from build123d import *

# Parameters (mm, degrees)
EXTRU_MINCE1_DEPTH      = 16.5
ENL_V_MAT_EXTRU_5_DEPTH = 37.379072455
BOSS_EXTRU_1_DEPTH      = 5
ESQUISSE2_R             = 1.6
ENL_V_MAT_EXTRU_1_DEPTH = 23.509707076
ESQUISSE3_R             = 1.6
ENL_V_MAT_EXTRU_2_DEPTH = 23.509707076
ENL_V_START             = -3
ENL_V_MAT_EXTRU_3_DEPTH = 20.509707076
ENL_V_MAT_EXTRU_4_DEPTH = 20.509707076
CHANFREIN1_SIZE         = 10
CONG_1_R                = 2


with BuildPart() as part:
    # Esquisse1 → Extru.-Mince1 (new, symmetric)
    with BuildSketch(Plane(origin=(0, 0, 0), x_dir=(0, 0, -1), z_dir=(1, 0, 0))):
        Polygon((11, 0), (0, 0), (-8.191520443, -5.735764364), (-4.750061825, -10.650676629), (1.891792733, -6), (11, -6), align=None)
    extrude(amount=EXTRU_MINCE1_DEPTH, both=True)

    # Esquisse7 → Enlèv. mat.-Extru.5 (cut, through all)
    with BuildSketch(Plane.ZY.offset(16.5)):
        Polygon((-1.891792733, -6), (5.081994449, -6), (7.04436757, -7.374068452), (4.750061825, -10.650676629), align=None)
    extrude(amount=-ENL_V_MAT_EXTRU_5_DEPTH, mode=Mode.SUBTRACT)

    # Esquisse6 → Boss.-Extru.1 (add, symmetric)
    with BuildSketch(Plane(origin=(0, 0, 0), x_dir=(0, 0, -1), z_dir=(1, 0, 0))):
        Polygon((1.891792733, -6), (11, -6), (-4.750061825, -10.650676629), (-8.191520443, -5.735764364), (-5.081994449, -6), align=None)
    extrude(amount=BOSS_EXTRU_1_DEPTH, both=True)

    # Esquisse2 → Enlèv. mat.-Extru.1 (cut, through all)
    with BuildSketch(Plane(origin=(0, 0, 0), x_dir=(1, 0, 0), z_dir=(0, 1, 0))):
        with Locations(Location((-12, 6.5, 0), (0, 0, 270))):
            Circle(ESQUISSE2_R)
        with Locations(Location((12, 6.5, 0), (0, 0, 90))):
            Circle(ESQUISSE2_R)
    extrude(amount=-ENL_V_MAT_EXTRU_1_DEPTH, mode=Mode.SUBTRACT)

    # Esquisse3 → Enlèv. mat.-Extru.2 (cut, through all)
    with BuildSketch(Plane(origin=(0, 0, 0), x_dir=(1, 0, 0), z_dir=(0, 0.819152044288991, 0.5735764363510473))):
        with Locations(Location((0, -5.5, 0), (0, 0, 270))):
            Circle(ESQUISSE3_R)
    extrude(amount=-ENL_V_MAT_EXTRU_2_DEPTH, mode=Mode.SUBTRACT)

    # Esquisse4 → Enlèv. mat.-Extru.3 (cut, through all)
    with BuildSketch(Plane(origin=(0, 0, 0), x_dir=(1, 0, 0), z_dir=(0, 1, 0)).offset(ENL_V_START)):
        Polygon((-9.25, 8.08771324), (-12, 9.675426481), (-14.75, 8.08771324), (-14.75, 4.91228676), (-12, 3.324573519), (-9.25, 4.91228676), align=None)
        Polygon((14.75, 8.08771324), (12, 9.675426481), (9.25, 8.08771324), (9.25, 4.91228676), (12, 3.324573519), (14.75, 4.91228676), align=None)
    extrude(amount=-ENL_V_MAT_EXTRU_3_DEPTH, mode=Mode.SUBTRACT)

    # Esquisse5 → Enlèv. mat.-Extru.4 (cut, through all)
    with BuildSketch(Plane(origin=(0, 0, 0), x_dir=(1, 0, 0), z_dir=(0, 0.819152044288991, 0.5735764363510474)).offset(ENL_V_START)):
        Polygon((2.75, -3.91228676), (0, -2.324573519), (-2.75, -3.91228676), (-2.75, -7.08771324), (0, -8.675426481), (2.75, -7.08771324), align=None)
    extrude(amount=-ENL_V_MAT_EXTRU_4_DEPTH, mode=Mode.SUBTRACT)

    # Chanfrein1
    chanfrein1_edges = [part.edges().sort_by_distance(p)[0] for p in [
        (-16.5, -6.554916408, 7.617944007),
        (16.5, -6.554916408, 7.617944007),
    ]]
    chamfer(chanfrein1_edges, length=CHANFREIN1_SIZE)

    # Congé1
    # the kernel refuses this fillet: 2 mm, written as the material it adds along each edge
    with BuildSketch(Plane(origin=(7, -8, 4.451396871), x_dir=(0, 0.819152044288991, 0.5735764363510474), z_dir=(-1, 0, 0))) as cong_1_piece_1_section:
        Polygon((0, 0), (CONG_1_R, 0), (CONG_1_R, CONG_1_R * 0.315298788879), (CONG_1_R * 0.819152044289, CONG_1_R * 0.573576436351), align=None)
    cong_1_piece_1 = extrude(amount=CONG_1_R, mode=Mode.PRIVATE)
    cong_1_piece_1 = cong_1_piece_1 - Plane(origin=(7, -8, 4.451396871), x_dir=(0, -0.9537169507482266, -0.30070579950427384), z_dir=(-1, 0, 0)) * Sphere(CONG_1_R, mode=Mode.PRIVATE)
    add(cong_1_piece_1)
    with BuildSketch(Plane(origin=(-7, -8, 4.451396871), x_dir=(0, 1, 0), z_dir=(1, 0, 0))) as cong_1_piece_2_section:
        Polygon((0, 0), (CONG_1_R, 0), (CONG_1_R, CONG_1_R * 0.315298788879), (CONG_1_R * 0.819152044289, CONG_1_R * 0.573576436351), align=None)
    cong_1_piece_2 = extrude(amount=CONG_1_R, mode=Mode.PRIVATE)
    cong_1_piece_2 = cong_1_piece_2 - Plane(origin=(-7, -8, 4.451396871), x_dir=(0, -0.9537169507482266, -0.30070579950427384), z_dir=(1, 0, 0)) * Sphere(CONG_1_R, mode=Mode.PRIVATE)
    add(cong_1_piece_2)
    with BuildSketch(Plane(origin=(7, -6, 5.081994449), x_dir=(0, 0, -1), z_dir=(1, 0, 0))) as cong_1_piece_3_section:
        with BuildLine():
            CenterArc((CONG_1_R * 0.315298788879, -CONG_1_R), CONG_1_R, 90, 35)
            Line((-CONG_1_R * 0.258277647472, -CONG_1_R * 0.180847955711), (0, 0))
            Line((0, 0), (CONG_1_R * 0.315298788879, 0))
        make_face()
    cong_1_piece_3 = extrude(amount=3.472109184, mode=Mode.PRIVATE)
    cong_1_piece_3 = split(cong_1_piece_3, bisect_by=Plane(origin=(8.435798526, -6.333350621, 5.409912391), z_dir=(-0.7071067811865476, 0.40557978767263964, -0.5792279653395686)), keep=Keep.TOP, mode=Mode.PRIVATE)
    add(cong_1_piece_3)
    with BuildSketch(Plane(origin=(-10.472109184, -6, 5.081994449), x_dir=(0, 0, -1), z_dir=(1, 0, 0))) as cong_1_piece_4_section:
        with BuildLine():
            CenterArc((CONG_1_R * 0.315298788879, -CONG_1_R), CONG_1_R, 90, 35)
            Line((-CONG_1_R * 0.258277647472, -CONG_1_R * 0.180847955711), (0, 0))
            Line((0, 0), (CONG_1_R * 0.315298788879, 0))
        make_face()
    cong_1_piece_4 = extrude(amount=3.472109184, mode=Mode.PRIVATE)
    cong_1_piece_4 = split(cong_1_piece_4, bisect_by=Plane(origin=(-8.435798526, -6.333350621, 5.409912391), z_dir=(0.7071067811865476, 0.40557978767263964, -0.5792279653395686)), keep=Keep.TOP, mode=Mode.PRIVATE)
    add(cong_1_piece_4)
    with BuildSketch(Plane(origin=(-5, -7.374068452, 7.04436757), x_dir=(-1, 0, 0), z_dir=(0, 0.5735764363510474, -0.819152044288991))) as cong_1_piece_5_section:
        with BuildLine():
            CenterArc((CONG_1_R, -CONG_1_R), CONG_1_R, 90, 90)
            Line((0, -CONG_1_R), (0, 0))
            Line((0, 0), (CONG_1_R, 0))
        make_face()
    cong_1_piece_5 = extrude(amount=1.765017662, mode=Mode.PRIVATE)
    cong_1_piece_5 = split(cong_1_piece_5, bisect_by=Plane(origin=(-6.416553747, -7.794178032, 6.852072741), z_dir=(0.7071067811865476, 0.40557978767263964, -0.5792279653395686)), keep=Keep.TOP, mode=Mode.PRIVATE)
    add(cong_1_piece_5)
    with BuildSketch(Plane(origin=(5, -7.374068452, 7.04436757), x_dir=(1, 0, 0), z_dir=(0, 0.5735764363510474, -0.819152044288991))) as cong_1_piece_6_section:
        with BuildLine():
            CenterArc((CONG_1_R, CONG_1_R), CONG_1_R, 180, 90)
            Line((0, CONG_1_R), (0, 0))
            Line((0, 0), (CONG_1_R, 0))
        make_face()
    cong_1_piece_6 = extrude(amount=1.765017662, mode=Mode.PRIVATE)
    cong_1_piece_6 = split(cong_1_piece_6, bisect_by=Plane(origin=(6.416553747, -7.794178032, 6.852072741), z_dir=(-0.7071067811865476, 0.40557978767263964, -0.5792279653395686)), keep=Keep.TOP, mode=Mode.PRIVATE)
    add(cong_1_piece_6)
    with BuildSketch(Plane(origin=(5, -6, 4.451396871), x_dir=(1, 0, 0), z_dir=(0, 0, -1))) as cong_1_piece_7_section:
        with BuildLine():
            CenterArc((CONG_1_R, CONG_1_R), CONG_1_R, 180, 90)
            Line((0, CONG_1_R), (0, 0))
            Line((0, 0), (CONG_1_R, 0))
        make_face()
    cong_1_piece_7 = extrude(amount=15.451396871, mode=Mode.PRIVATE)
    cong_1_piece_7 = split(cong_1_piece_7, bisect_by=Plane(origin=(5.479319135, -8.319320936, -3.145347646), z_dir=(0, 0.9590632108966768, 0.2831920858791019)), keep=Keep.TOP, mode=Mode.PRIVATE)
    add(cong_1_piece_7)
    with BuildSketch(Plane(origin=(-5, -6, -11), x_dir=(-1, 0, 0), z_dir=(0, 0, 1))) as cong_1_piece_8_section:
        with BuildLine():
            CenterArc((CONG_1_R, CONG_1_R), CONG_1_R, 180, 90)
            Line((0, CONG_1_R), (0, 0))
            Line((0, 0), (CONG_1_R, 0))
        make_face()
    cong_1_piece_8 = extrude(amount=15.451396871, mode=Mode.PRIVATE)
    cong_1_piece_8 = split(cong_1_piece_8, bisect_by=Plane(origin=(-5.479319135, -8.319320936, -3.145347646), z_dir=(0, 0.9590632108966768, 0.2831920858791019)), keep=Keep.TOP, mode=Mode.PRIVATE)
    add(cong_1_piece_8)
    # the kernel refuses this fillet: 2 mm, written as the material it takes off along each edge
    with BuildSketch(Plane(origin=(-16.5, 1.696519432, 1.187915695), x_dir=(0, 0.5735764363510472, -0.8191520442889909), z_dir=(0, -0.819152044288991, -0.5735764363510473)), Plane(origin=(16.5, 1.696519432, 1.187915695), x_dir=(-0.7071067811865467, -0.40557978767264014, 0.5792279653395693), z_dir=(0, -0.819152044288991, -0.5735764363510473))) as cong_1_2_piece_1:
        with BuildLine():
            CenterArc((CONG_1_R * 0.414213562373, CONG_1_R), CONG_1_R, 225, 45)
            Line((-CONG_1_R * 0.292893218813, CONG_1_R * 0.292893218813), (0, 0))
            Line((0, 0), (CONG_1_R * 0.414213562373, 0))
        make_face()
    extrude(amount=11.466783156, mode=Mode.SUBTRACT)
    with BuildSketch(Plane(origin=(6.5, -9.12261086, 5.820024995), x_dir=(-1, 0, 0), z_dir=(0, 0.8191520442889916, 0.5735764363510465))) as cong_1_2_piece_2:
        with BuildLine():
            CenterArc((CONG_1_R * 0.414213562373, -CONG_1_R), CONG_1_R, 90, 45)
            Line((-CONG_1_R * 0.292893218813, -CONG_1_R * 0.292893218813), (0, 0))
            Line((0, 0), (CONG_1_R * 0.414213562373, 0))
        make_face()
    extrude(amount=6.205643951, mode=Mode.SUBTRACT)
    with BuildSketch(Plane(origin=(-6.5, -9.12261086, 5.820024995), x_dir=(1, 0, 0), z_dir=(-1.721686136418026e-15, 0.8191520442889914, 0.5735764363510468))) as cong_1_2_piece_3:
        with BuildLine():
            CenterArc((CONG_1_R * 0.414213562373, CONG_1_R), CONG_1_R, 225, 45)
            Line((-CONG_1_R * 0.292893218813, CONG_1_R * 0.292893218813), (0, 0))
            Line((0, 0), (CONG_1_R * 0.414213562373, 0))
        make_face()
    extrude(amount=6.205643951, mode=Mode.SUBTRACT)
    with BuildSketch(Plane(origin=(16.5, -11, -11), x_dir=(0, 0, 1), z_dir=(0, 1, 0))) as cong_1_2_piece_4:
        with BuildLine():
            CenterArc((CONG_1_R, -CONG_1_R), CONG_1_R, 90, 90)
            Line((0, -CONG_1_R), (0, 0))
            Line((0, 0), (CONG_1_R, 0))
        make_face()
    extrude(amount=16, mode=Mode.SUBTRACT)
    with BuildSketch(Plane(origin=(8.596227372, -10.650676629, 4.750061825), x_dir=(0, 0.2831920858791011, -0.9590632108966769), z_dir=(-1, 0, 0))) as cong_1_2_piece_5:
        with BuildLine():
            CenterArc((CONG_1_R * 0.719245474399, -CONG_1_R), CONG_1_R, 90, 71.450811124)
            Line((-CONG_1_R * 0.22880542283, -CONG_1_R * 0.681881317333), (0, 0))
            Line((0, 0), (CONG_1_R * 0.719245474399, 0))
        make_face()
    extrude(amount=17.192454744, mode=Mode.SUBTRACT)
    with BuildSketch(Plane(origin=(-16.5, -11, -11), x_dir=(0, 0, 1), z_dir=(0, 1, 0))) as cong_1_2_piece_6:
        with BuildLine():
            CenterArc((CONG_1_R, CONG_1_R), CONG_1_R, 180, 90)
            Line((0, CONG_1_R), (0, 0))
            Line((0, 0), (CONG_1_R, 0))
        make_face()
    extrude(amount=16, mode=Mode.SUBTRACT)


solid = part.part
Build history of the part. All positions in model axes, mm. A direction names the side the tool comes from. Round coordinates to 2 decimals unless told otherwise and drop trailing zeros. Loops run counter-clockwise (first coordinate to the right, second up) from the corner with the lowest first, then second, coordinate; pieces in that order, holes last. Notation, with made-up numbers: (41.5, 51.25) -> (55.5, 51.25) arc R22 ccw to (55.5, 82.25) -> close; hole circle Ø3 at (10.25, -20). An arc over 180 degrees is marked (long way). Answer in a Markdown table with one row per item.
Item 1: Pin check, flat tips, straight feed: pin 1 (1.9 mm diameter, centred on y = -9.5, z = -0.5, fed in from +X); pin 2 (10.5 mm diameter, centred on x = -9.5, z = -5.5, fed in from -Y); pin 3 (3 mm diameter, centred on x = 10.5, z = -3, fed in from -Y); pin 4 (1.9 mm diameter, centred on x = -12, z = -6.5, fed in from +Y). Stop position of each tip, or through.
Answers below:
| item | result |
|---|---|
| pin 1 | stops at x = 5 |
| pin 2 | stops at y = -8.42 |
| pin 3 | stops at y = -6 |
| pin 4 | passes through |
Item 2: Drill centre lines: L1, parallel to X at y = -2.3, z = -6.5; L2, parallel to X at y = -5.5, z = -9.25; L3, parallel to Z at x = 12, y = -1.85. Where is each one in solid material? Low to high. Write a range as [from, to].
Answers below:
| item | result |
|---|---|
| L1 | x = [-16.5, -13.6], [-10.4, 10.4], [13.6, 16.5] |
| L2 | x = [-16.48, -12.74], [-11.26, 11.26], [12.74, 16.48] |
| L3 | z = [-11, -8.1], [-4.9, 2.64] |
Item 3: Saw through at D-D (x = 14). Write the cut outline in (y, z).
Answers below:
| item | result |
|---|---|
| outline | (-6, -11) -> (0, -11) -> (0, 0) -> (-1.43, 2.05) -> (-6, -1.15) -> (-6, -4.48) -> (-3, -4.48) -> (-3, -8.52) -> (-6, -8.52) -> close |
Item 4: Mould opens along X. For faces 1 (the flat face through (7.483, -6.638, 5.993)), 2 (the cylindrical face through (13.42, -1.48, -7.24)), 3 (the cylindrical face through (-5.6, -7.34, 6)) say: +X half, -X half, draft (parallel to the pull), parting line (faces both ways), or undercut.
Answers below:
| item | result |
|---|---|
| face 1 | draft |
| face 2 | undercut |
| face 3 | -X half |
Item 5: Which spindle directions (+Z, -Z, +X, -X, +Y, -Y) get a long thin tool onto all of the face, cutting with end or side? Do faces 4 (the flat face through (0.228, -1.553, 2.218)), 5 (the cylindrical face through (15.93, -3.04, -10.4)), 6 (the cylindrical face through (-7.95, -6.09, 5.04)), 7 (the flat face through (10.606, -4.479, -4.13)), 8 (the flat face through (-2.75, -8, 1)). Say none if no direction does.
Answers below:
| item | result |
|---|---|
| face 4 | +Z, +X, -X, +Y |
| face 5 | -Z, +X, +Y, -Y |
| face 6 | -Z, -X, -Y |
| face 7 | -Y |
| face 8 | none |
Item 6: Saw through at C-C (y = -1.25). State how many separate pieces and enclosed holes the cut face has, and give its area (3 significant figures).
Answers below:
| item | result |
|---|---|
| separate pieces | 1 |
| enclosed holes | 2 |
| area | 398 mm² |
Item 7: Saw through at B-B (x = 4). Write the cut outline in (y, z).
Answers below:
| item | result |
|---|---|
| outline | (-10.24, 3.37) -> (-6, -11) -> (0, -11) -> (0, 0) -> (-5.74, 8.19) -> (-9.47, 5.58) arc R2 ccw to start |
Item 8: Saw through at A-A (z = -6.5). Write the cut outline in (x, y).
Answers below:
| item | result |
|---|---|
| outline | (-16.5, -6) -> (-14.75, -6) -> (-14.75, -3) -> (-13.6, -3) -> (-13.6, 0) -> (-16.5, 0) -> close; (-10.4, -3) -> (-9.25, -3) -> (-9.25, -6) -> (-7, -6) arc R2 cw to (-5.12, -7.33) -> (5.12, -7.33) arc R2 cw to (7, -6) -> (9.25, -6) -> (9.25, -3) -> (10.4, -3) -> (10.4, 0) -> (-10.4, 0) -> close; (13.6, -3) -> (14.75, -3) -> (14.75, -6) -> (16.5, -6) -> (16.5, 0) -> (13.6, 0) -> close |
